Job drawing, mm, ordinate dimensions from the low corner. One solid piece. Give positions to 0.01 mm unless a question says otherwise; leave off trailing zeros. Write each loop counter-clockwise with the first axis right and the second up, starting at its lowest first coordinate (ties: lowest second). Pieces come first, ordered by that corner, then holes. Notation, with made-up numbers: M -26,59 L -10,59 A32 cw -10,93 Z; hole C 33,71.5 d11. An arc over 180 degrees is marked long. Use CSV: the item, a comma, the result in double quotes. Start each with the question number.
Item 1: Pin check, flat tips, straight feed: pin 1 (4 mm diameter, centred on x = 48.53, z = 49.93, fed in from +Y); pin 2 (1.5 mm diameter, centred on x = 99.5, y = 7.5, fed in from -Z); pin 3 (4 mm diameter, centred on x = 111, y = 8.5, fed in from +Z). Stop position of each tip, or through.
Item 2: Cut at A-A (z = 80). List the corners of the cut face in (x, y).
Item 3: Cut at B-B (y = 7.25). List the corners of the cut face in (x, z).
Item 4: Mould opens along X. For the marked faces 1 and 2 say: released by +X, released by -X, zero draft, split by the parting line, or undercut.
Item 5: Cut at C-C (x = 78.5). List the corners of the cut face in (y, z).
Item 6: Drill centre lines: line 1 (X direction, y = 8, z = 44); line 2 (Z direction, x = 34.5, y = 8); line 3 (Y direction, x = 76, z = 51). Where is each one in solid material? Low to high. Write a range as [from, to].
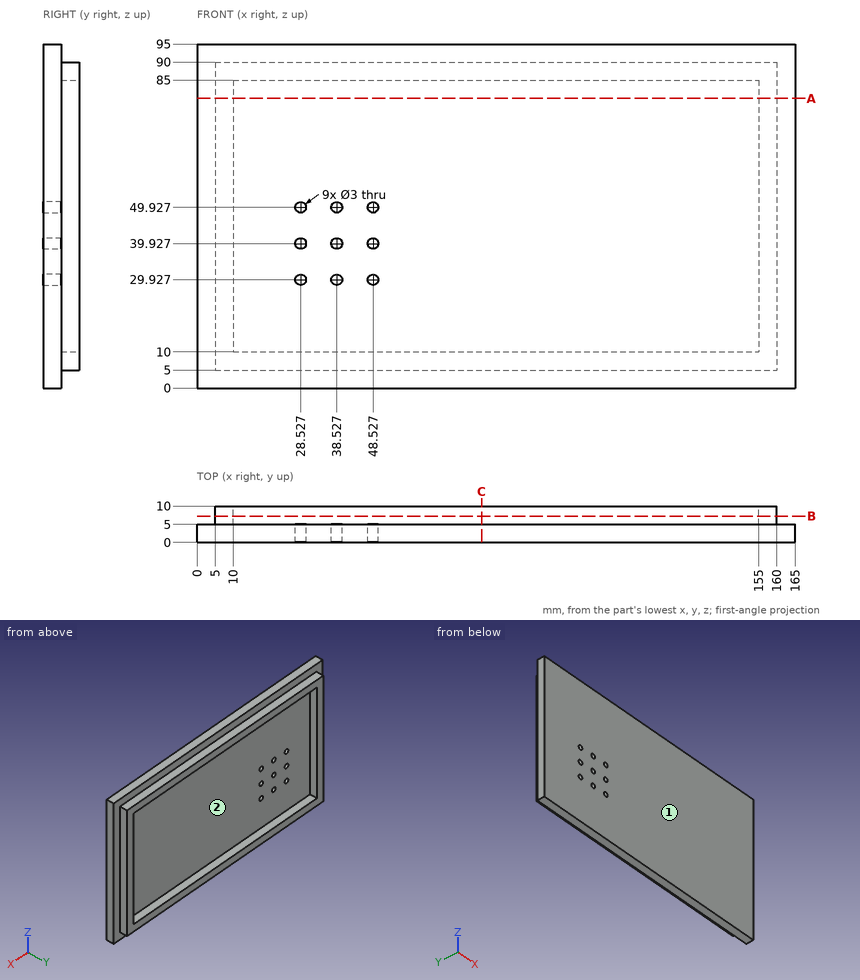
Worked answers:
1,pin 1,"stops at y = 5"
1,pin 2,"stops at z = 5"
1,pin 3,"stops at z = 90"
2,outline,"M 0,0 L 165,0 L 165,5 L 160,5 L 160,10 L 155,10 L 155,5 L 10,5 L 10,10 L 5,10 L 5,5 L 0,5 Z"
3,outline,"M 5,5 L 160,5 L 160,90 L 5,90 Z; hole M 10,10 L 155,10 L 155,85 L 10,85 Z"
4,face 1,"zero draft"
4,face 2,"undercut"
5,outline,"M 0,0 L 5,0 L 5,5 L 10,5 L 10,10 L 5,10 L 5,85 L 10,85 L 10,90 L 5,90 L 5,95 L 0,95 Z"
6,line 1,"x = [5, 10], [155, 160]"
6,line 2,"z = [5, 10], [85, 90]"
6,line 3,"y = [0, 5]"
